The model under review builds one solid part; all positions refer to its coordinate system, in mm. A direction names the side the tool comes from. Coordinates: 2 decimals unless noted, no trailing zeros. Order: outer loops, then holes, each group sorted by start corner. A loop starts at its lowest first (then second) coordinate and runs counter-clockwise, first axis right, second up. Notation, with made-up numbers: (-37, -18) - (19, -18) arc R27 cw to (19, 10) - close; hole circle Ø1 at (72, 55). An arc over 180 degrees is marked (long way). Answer in a Markdown table with one row per item.
```python
from build123d import *

# Parameters (mm, degrees)
W_TOP_DEPTH         = 3.175
SKETCH3_W           = 35.6
SKETCH3_H           = 4.6
SKETCH3_W_2         = 16.4
SKETCH3_H_2         = 12
A_HOLDERS_DEPTH     = 5.5
HOLDER_CHAMFER_R    = 1.25
A_CLAMP_DEPTH       = 2
SKETCH12_R          = 1.35
SKETCH12_W          = 25
SKETCH12_H          = 45.3
A_HOLES_DEPTH       = 3.175
A_HOLES_GUIDE_DEPTH = 1.5
SKETCH15_R          = 3.225
TENDON_HOLES_DEPTH  = 3.175


with BuildPart() as part:
    # Sketch1 → w_top (new body)
    with BuildSketch(Plane(origin=(0, 0, 0), x_dir=(1, 0, 0), z_dir=(0, 1, 0))):
        with BuildLine():
            Line((-48, -35), (-48, 30))
            ThreePointArc((-48, 30), (-42.142135624, 44.142135624), (-28, 50))
            Line((-28, 50), (28, 50))
            ThreePointArc((28, 50), (42.142135624, 44.142135624), (48, 30))
            Line((48, 30), (48, -35))
            ThreePointArc((48, -35), (42.142135624, -49.142135624), (28, -55))
            Line((28, -55), (-28, -55))
            ThreePointArc((-28, -55), (-42.142135624, -49.142135624), (-48, -35))
        make_face()
    extrude(amount=W_TOP_DEPTH)

    # Sketch3 → a_holders (add)
    with BuildSketch(Plane(origin=(0, 3.175, 0), x_dir=(1, 0, 0), z_dir=(0, 1, 0))):
        Polygon((-33, 22), (-33, 38), (-8.6, 38), (-8.6, 22), (8.6, 22), (8.6, 38), (33, 38), (33, 22), (41.1, 22), (41.1, 12.5), (-41.1, 12.5), (-41.1, 22), align=None)
        with Locations((20.8, 17.3)):
            Rectangle(SKETCH3_W, SKETCH3_H, mode=Mode.SUBTRACT)
        with Locations((-20.8, 17.3)):
            Rectangle(SKETCH3_W, SKETCH3_H, mode=Mode.SUBTRACT)
        with Locations((-20.8, 28)):
            Rectangle(SKETCH3_W_2, SKETCH3_H_2, mode=Mode.SUBTRACT)
        with Locations((20.8, 28)):
            Rectangle(SKETCH3_W_2, SKETCH3_H_2, mode=Mode.SUBTRACT)
        Polygon((8.6, -22), (0.5, -22), (0.5, -12.5), (41.1, -12.5), (41.1, -22), (33, -22), (33, -38), (8.6, -38), align=None)
        with Locations((20.8, -17.3)):
            Rectangle(SKETCH3_W, SKETCH3_H, mode=Mode.SUBTRACT)
        with Locations((20.8, -28)):
            Rectangle(SKETCH3_W_2, SKETCH3_H_2, mode=Mode.SUBTRACT)
    extrude(amount=A_HOLDERS_DEPTH)

    # holder_chamfer
    holder_chamfer_edges = [part.edges().sort_by_distance(p)[0] for p in [
        (0.5, 3.175, 17.25),
        (20.8, 3.175, 12.5),
        (41.1, 3.175, 17.25),
        (37.05, 3.175, 22),
        (33, 3.175, 30),
        (20.8, 3.175, 38),
        (8.6, 3.175, 30),
        (4.55, 3.175, 22),
        (41.1, 3.175, -17.25),
        (0, 3.175, -12.5),
        (-41.1, 3.175, -17.25),
        (-37.05, 3.175, -22),
        (-33, 3.175, -30),
        (-20.8, 3.175, -38),
        (-8.6, 3.175, -30),
        (0, 3.175, -22),
        (8.6, 3.175, -30),
        (20.8, 3.175, -38),
        (33, 3.175, -30),
        (37.05, 3.175, -22),
    ]]
    fillet(holder_chamfer_edges, radius=HOLDER_CHAMFER_R)

    # Sketch14 → a_clamp (add)
    with BuildSketch(Plane(origin=(0, 8.675, 0), x_dir=(1, 0, 0), z_dir=(0, 1, 0))):
        Polygon((-35.6, 19.6), (-35.6, 22), (-41.1, 22), (-41.1, 12.5), (-35.6, 12.5), (-35.6, 15), (-38.6, 15), (-38.6, 19.6), align=None)
        Polygon((-3, 19.6), (-6, 19.6), (-6, 22), (6, 22), (6, 19.6), (3, 19.6), (3, 15), (6, 15), (6, 12.5), (-6, 12.5), (-6, 15), (-3, 15), align=None)
        Polygon((38.6, 19.6), (35.6, 19.6), (35.6, 22), (41.1, 22), (41.1, 12.5), (35.6, 12.5), (35.6, 15), (38.6, 15), align=None)
        Polygon((0.5, -12.5), (6, -12.5), (6, -15), (3, -15), (3, -19.6), (6, -19.6), (6, -22), (0.5, -22), align=None)
        Polygon((35.6, -19.6), (35.6, -22), (41.1, -22), (41.1, -12.5), (35.6, -12.5), (35.6, -15), (38.6, -15), (38.6, -19.6), align=None)
    extrude(amount=A_CLAMP_DEPTH)

    # Sketch12 → a_holes (cut)
    with BuildSketch(Plane(origin=(0, 3.175, 0), x_dir=(1, 0, 0), z_dir=(0, 1, 0))):
        with Locations((-28.8, -47.8)):
            Circle(SKETCH12_R)
        with Locations((-11.8, -47.8)):
            Circle(SKETCH12_R)
        with Locations((-35.3, -24.5)):
            Circle(SKETCH12_R)
        with Locations((-5.3, -24.5)):
            Circle(SKETCH12_R)
        with Locations((-20.3, -22.45)):
            Rectangle(SKETCH12_W, SKETCH12_H)
    extrude(amount=-A_HOLES_DEPTH, mode=Mode.SUBTRACT)

    # Sketch13 → a_holes guide (cut)
    with BuildSketch(Plane.XZ):
        with BuildLine():
            Line((-31.6, 47.8), (-31.6, 45.1))
            Line((-31.6, 45.1), (-26, 45.1))
            Line((-26, 45.1), (-26, 47.8))
            ThreePointArc((-26, 47.8), (-28.8, 50.6), (-31.6, 47.8))
        make_face()
        with BuildLine():
            Line((-35.3, 27.3), (-32.8, 27.3))
            Line((-32.8, 27.3), (-32.8, 21.7))
            Line((-32.8, 21.7), (-35.3, 21.7))
            ThreePointArc((-35.3, 21.7), (-38.1, 24.5), (-35.3, 27.3))
        make_face()
        with BuildLine():
            Line((-7.8, 21.7), (-5.3, 21.7))
            ThreePointArc((-5.3, 21.7), (-2.5, 24.5), (-5.3, 27.3))
            Line((-5.3, 27.3), (-7.8, 27.3))
            Line((-7.8, 27.3), (-7.8, 21.7))
        make_face()
        with BuildLine():
            Line((-14.6, 45.1), (-14.6, 47.8))
            ThreePointArc((-14.6, 47.8), (-11.8, 50.6), (-9, 47.8))
            Line((-9, 47.8), (-9, 45.1))
            Line((-9, 45.1), (-14.6, 45.1))
        make_face()
    extrude(amount=-A_HOLES_GUIDE_DEPTH, mode=Mode.SUBTRACT)

    # Sketch15 → tendon holes (cut)
    with BuildSketch(Plane(origin=(0, 3.175, 0), x_dir=(1, 0, 0), z_dir=(0, 1, 0))):
        with Locations((-31.3, 6.33)):
            Circle(SKETCH15_R)
        with Locations((31.3, 6.33)):
            Circle(SKETCH15_R)
        with Locations((31.3, -6.33)):
            Circle(SKETCH15_R)
    extrude(amount=-TENDON_HOLES_DEPTH, mode=Mode.SUBTRACT)


solid = part.part
```
Item 1: To check wall thickness, follow line 1 (Z direction, x = 17, y = 4.25); line 2 (Z direction, x = -17, y = 5.5); line 3 (Z direction, x = -5.3, y = 2). State the ranges of each line that lie inside material, in increasing order. Write a range as from..to.
Check values:
| item | result |
|---|---|
| line 1 | -38.01..-34, -22..-19.6, -15..-12.49, 12.49..15, 19.6..22, 34..38.01 |
| line 2 | -38..-34, -22..-19.6, -15..-12.5 |
| line 3 | -50..23.15, 25.85..55 |
Item 2: Tool access review of faces 1 (the face through (-11.9, 0.7, 50.6)), 2 (the face through (-21, 8.675, -35)), 3 (the face through (21, 6, -15)): name each direction out of +Z, -Z, +X, -X, +Y, -Y from which nothing blocks a thin tool from reaching the whole face with its end or side.
Check values:
| item | result |
|---|---|
| face 1 | -Y |
| face 2 | +Z, -Z, +Y |
| face 3 | +Y |
Item 3: Clearance check with flat-ended pins moving along their axes: pin 1 Ø2 at (x, y) = (-19, 6) entering from -Z; pin 2 Ø1.2 at (x, y) = (-33.5, 0.5) entering from +Z; pin 3 Ø1.3 at (y, z) = (6, -27.5) entering from +X. State where each tip first meets the part, or that it passes through.
Check values:
| item | result |
|---|---|
| pin 1 | z = -38 |
| pin 2 | z = 54.39 |
| pin 3 | x = 33 |
Item 4: Mouldability with a two-part tool opening along X and no side actions: class faces 4 (the face through (0, 2, 55)), 5 (the face through (33, 7, -30)), 6 (the face through (-27.6, 1.5, 46.7)) as +X half, -X half, draft (parallel to the pull), parting line (faces both ways), or undercut.
Check values:
| item | result |
|---|---|
| face 4 | draft |
| face 5 | +X half |
| face 6 | undercut |
Item 5: We need section B-B, the plane z = -6.33. Write out the cut boundary in (x, y) (3 decimals), then the cut area to 3 significant figures.
Check values:
| item | result |
|---|---|
| outline | (-48, 0) - (-34.525, 0) - (-34.525, 3.175) - (-48, 3.175) - close; (-28.075, 0) - (28.075, 0) - (28.075, 3.175) - (-28.075, 3.175) - close; (34.525, 0) - (48, 0) - (48, 3.175) - (34.525, 3.175) - close |
| area | 264 mm^2 |
Item 6: We need section A-A, the plane z = 24.5. State how many separate pieces and enclosed holes the cut face has, then the cut area to 3 significant figures.
Check values:
| item | result |
|---|---|
| separate pieces | 4 |
| enclosed holes | 0 |
| area | 245 mm^2 |
Item 7: We need section C-C, the plane x = -22. Write out the cut boundary in (y, z) (3 decimals).
Check values:
| item | result |
|---|---|
| outline | (0, -50) - (3.175, -50) - (3.175, -39.25) arc R1.25 cw to (4.425, -38) - (8.675, -38) - (8.675, -34) - (3.175, -34) - (3.175, -22) - (8.675, -22) - (8.675, -19.6) - (3.175, -19.6) - (3.175, -15) - (8.675, -15) - (8.675, -12.5) - (4.425, -12.5) arc R1.25 cw to (3.175, -11.25) - (3.175, -0.2) - (0, -0.2) - close; (0, 45.1) - (3.175, 45.1) - (3.175, 55) - (0, 55) - close |
